The listing builds one solid part. Answer for the finished solid, in the listing's coordinates (mm). A direction names the side the tool comes from. Give positions to 0.01 mm unless a question says otherwise; leave off trailing zeros. Write each loop counter-clockwise with the first axis right and the second up, starting at its lowest first coordinate (ties: lowest second). Pieces come first, ordered by that corner, then holes. Notation, with made-up numbers: M -5,59.5 L 52,59.5 A14 ccw 52,71.5 Z; hole C 87,43 d8. An arc over 180 degrees is marked long. Answer as a JSON object with one key per item and string values.
```python
from build123d import *

# Parameters (mm, degrees)
SKETCH1_R             = 5
BASE_DEPTH            = 22
SKETCH2_W             = 27.5
SKETCH2_H             = 14.5
WIRE_INSERTIONS_DEPTH = 1.8
SKETCH3_R             = 1.5
GND_WIRES_DEPTH       = 25
SKETCH4_R             = 1.5
OUTPUT_WIRE_DEPTH     = 25
SKETCH5_R             = 1.5
INPUT_WIRE_DEPTH      = 25


with BuildPart() as part:
    # Sketch1 → Base (new body)
    with BuildSketch(Plane(origin=(0, 0, 0), x_dir=(1, 0, 0), z_dir=(0, 1, 0))):
        Polygon((22.25, -31.75), (-22.25, -31.75), (-28.75, -25.25), (-28.75, 25.25), (-22.25, 31.75), (22.25, 31.75), (28.75, 25.25), (28.75, -25.25), align=None)
        with Locations(Location((-3.75, -25.25, 0), (0, 0, 270))):
            Circle(SKETCH1_R, mode=Mode.SUBTRACT)
        with Locations(Location((-3.75, 25.25, 0), (0, 0, 270))):
            Circle(SKETCH1_R, mode=Mode.SUBTRACT)
    extrude(amount=BASE_DEPTH)

    # Sketch2 → Wire Insertions (add)
    with BuildSketch(Plane.ZY.offset(28.75)):
        with Locations((0, 7.25)):
            Rectangle(SKETCH2_W, SKETCH2_H)
    extrude(amount=WIRE_INSERTIONS_DEPTH)

    # Sketch3 → GND Wires (add)
    with BuildSketch(Plane.ZY.offset(30.55)):
        with Locations(Location((-2.25, 4, 0), (0, 0, 180))):
            Circle(SKETCH3_R)
        with Locations(Location((2.25, 4, 0), (0, 0, 180))):
            Circle(SKETCH3_R)
    extrude(amount=GND_WIRES_DEPTH)

    # Sketch4 → Output Wire (add)
    with BuildSketch(Plane.ZY.offset(30.55)):
        with Locations(Location((-6.75, 4, 0), (0, 0, 180))):
            Circle(SKETCH4_R)
    extrude(amount=OUTPUT_WIRE_DEPTH)

    # Sketch5 → Input Wire (add)
    with BuildSketch(Plane.ZY.offset(30.55)):
        with Locations(Location((6.75, 4, 0), (0, 0, 180))):
            Circle(SKETCH5_R)
    extrude(amount=INPUT_WIRE_DEPTH)


solid = part.part
```
1. A cutting plane is placed at A-A, the plane x = -3.75. Give the vertices of the cut face in (y, z).
Verdict:
{"outline": "M 0,-31.75 L 22,-31.75 L 22,-30.25 L 0,-30.25 Z; M 0,-20.25 L 22,-20.25 L 22,20.25 L 0,20.25 Z; M 0,30.25 L 22,30.25 L 22,31.75 L 0,31.75 Z"}
2. Consider line 1 along Z through (x, y) = (-38.5, 4); line 2 along X through (y, z) = (5.5, 25.25). Determine where each line is inside the solid, lowest interval first.
Verdict:
{"line 1": "z = -8.25 to -5.25, -3.75 to -0.75, 0.75 to 3.75, 5.25 to 8.25", "line 2": "x = -28.75 to -8.75, 1.25 to 28.75"}
3. For faces 4 (the flat face through (-28.75, 16, 0)), 5 (the flat face through (-55.55, 4, -7)), 6 (the cylindrical face through (-42.875, 2.735, 1.444)), determine the directions among +Z, -Z, +X, -X, +Y, -Y from which every point of the face is accessible in a straight line to the end or side of a thin tool.
Verdict:
{"face 4": "-X, +Y", "face 5": "+Z, -Z, -X, +Y, -Y", "face 6": "-X"}
4. A cutting plane is placed at C-C, the plane z = 2.25. Give the vertices of the cut face in (x, y).
Verdict:
{"outline": "M -55.55,2.5 L -30.55,2.5 L -30.55,0 L 28.75,0 L 28.75,22 L -28.75,22 L -28.75,14.5 L -30.55,14.5 L -30.55,5.5 L -55.55,5.5 Z"}
5. A cutting plane is placed at B-B, the plane y = 20.5. Give the vertices of the cut face in (x, z), plus the area to 3 significant figures.
Verdict:
{"outline": "M -28.75,-25.25 L -22.25,-31.75 L 22.25,-31.75 L 28.75,-25.25 L 28.75,25.25 L 22.25,31.75 L -22.25,31.75 L -28.75,25.25 Z; hole C -3.75,-25.25 d10; hole C -3.75,25.25 d10", "area": "3,410 mm2"}
6. Flat-ended cylindrical pins translate along their axes: pin 1 (2 mm diameter, centred on x = -30, y = 5.5, fed in from +Z); pin 2 (1.4 mm diameter, centred on x = -29.5, z = 0.5, fed in from +Y); pin 3 (11 mm diameter, centred on y = 10.5, z = 0, fed in from -X); pin 4 (12 mm diameter, centred on y = 12.5, z = 15.5, fed in from -X). Find the tip coordinate at first contact, or state that the pin passes through.
Verdict:
{"pin 1": "stops at z = 13.75", "pin 2": "stops at y = 14.5", "pin 3": "stops at x = -55.55", "pin 4": "stops at x = -30.55"}
7. The mould has two halves that part along Z. Classify faces 1 (the flat face through (-55.55, 4, -2)), 2 (the flat face through (-30, 7, -13.75)), 3 (the cylindrical face through (-42.88, 2.99, -1.14)): released by +Z, released by -Z, zero draft, split by the parting line, or undercut.
Verdict:
{"face 1": "zero draft", "face 2": "released by -Z", "face 3": "undercut"}
8. A cutting plane is placed at D-D, the plane y = 4. Count the separate pieces of the cut face and the enclosed holes in it, plus the area to 3 significant figures.
Verdict:
{"separate pieces": "1", "enclosed holes": "2", "area": "3,760 mm2"}
